Autodesk Inventor part; units mm, degrees
ref_plane "YZ Plane" through (0, 0, 0) normal (1, 0, 0) x (0, 1, 0)
ref_plane "XZ Plane" through (0, 0, 0) normal (0, 1, 0) x (-1, 0, 0)
ref_plane "XY Plane" through (0, 0, 0) normal (0, 0, 1) x (1, 0, 0)
sketch "Sketch1" plane through (0, 0, 0) normal (0, 0, 1) x (1, 0, 0)
  line L0 (6.5024, 2.8448) -> (6.5024, 17.6276)
  line L1 (6.5024, 17.6276) -> (-6.5024, 17.6276)
  line L2 (-6.5024, 2.8448) -> (-6.5024, 17.6276)
  circle A0 centre (0, 0) radius 3.5052 construction
  line L3 (0.1524, -3.5052) -> (-0.1524, -3.5052)
  arc A1 (-6.5024, 2.8448) -> (-0.1524, -3.5052) centre (-0.1524, 2.8448) ccw
  arc A2 (0.1524, -3.5052) -> (6.5024, 2.8448) centre (0.1524, 2.8448) ccw
  circle A3 centre (0, 0) radius 2.1844
  circle A4 centre (0, 0) radius 6.5024 construction
  dimension "d3" = 13.0048
  dimension "d5" = 7.0104
  dimension "d6" = 6.35
  dimension "d7" = 4.3688
  dimension "d10" = 13.0048
  dimension "d11" = 17.6276
extrude "Extrusion1" add sketch "Sketch1" along normal blind 20.32
sketch "Sketch2" plane through (6.5024, 2.8448, 0) normal (1, 0, 0) x (0, 0, -1)
  line L0 (-20.32, 0) -> (-20.32, 14.7828) construction
  line L1 (-20.32, 9.7028) -> (0, 9.7028) construction
  line L2 (0, 14.7828) -> (-20.32, 14.7828) construction
  line L3 (-20.32, 4.9276) -> (0, 4.9276) construction
  line L4 (0, 14.7828) -> (0, 0) construction
  line L5 (0, 0) -> (-20.32, 0) construction
  line L6 (0, -0.6604) -> (-20.32, -0.6604) construction
  line L7 (0, -5.0292) -> (-20.32, -5.0292) construction
  line L8 (0, -0.6604) -> (0, -5.0292) construction
  line L9 (0, -6.35) -> (0, 0) construction
  line L10 (-10.16, 14.7828) -> (-10.16, -6.35) construction
  line L11 (0, -6.35) -> (-20.32, -6.35) construction
  line L12 (-5.9055, 4.9276) -> (-5.9055, -6.35)
  line L13 (-5.9055, -6.35) -> (-10.16, -6.35)
  line L14 (-14.4145, 4.9276) -> (-14.4145, -6.35)
  line L15 (-14.4145, -6.35) -> (-10.16, -6.35)
  line L16 (-10.16, 9.7028) -> (-4.826, 9.7028)
  line L17 (-4.826, 9.7028) -> (-4.826, 4.9276)
  line L18 (-10.16, 9.7028) -> (-15.494, 9.7028)
  line L19 (-15.494, 9.7028) -> (-15.494, 4.9276)
  line L20 (-15.494, 4.9276) -> (-14.4145, 4.9276)
  line L21 (-4.826, 4.9276) -> (-5.9055, 4.9276)
  point P0 (0, -2.8448)
  dimension "d12" = 5.08
  dimension "d14" = 7.7724
  dimension "d15" = 4.2545
  dimension "d16" = 4.2545
extrude "Extrusion2" cut sketch "Sketch2" against normal through all
sketch "Sketch3" plane through (-6.5024, 17.6276, 0) normal (0, 1, 0) x (1, 0, 0)
  line L0 (6.6548, -14.4145) -> (6.6548, -20.32) construction
  line L1 (0, 0) -> (13.0048, 0) construction
  line L2 (6.5024, 0) -> (6.5024, -20.32) construction
  line L3 (13.0048, -20.32) -> (0, -20.32) construction
  line L4 (13.0048, 0) -> (13.0048, -20.32) construction
  line L5 (13.0048, -10.16) -> (0, -10.16) construction
  line L6 (0, 0) -> (0, -20.32) construction
  circle A0 centre (6.5024, -10.16) radius 1.9685 construction
  point P0 (6.5024, 0)
  dimension "d21" = 6.5024
  dimension "d22" = 10.16
  dimension "d23" = 3.937
hole "Hole1" at (0, 17.6276, 10.16) direction (0, -1, 0) diameter 3.937 end through all
sketch "Sketch4" plane through (0, 0, 20.32) normal (0, 0, 1) x (1, 0, 0)
  circle A0 centre (0, 0) radius 3.81
  dimension "d31" = 7.62
extrude "Extrusion3" cut sketch "Sketch4" against normal blind 2.54
sketch "Sketch5" plane through (0, 0, 0) normal (0, 0, -1) x (-1, 0, 0)
  circle A0 centre (0, 0) radius 2.1844 construction
  circle A1 centre (0, 0) radius 4.1275 construction
  line L0 (-4.1275, 0) -> (-2.0638, 3.5745)
  line L1 (-2.0638, 3.5745) -> (2.0637, 3.5745)
  line L2 (2.0637, 3.5745) -> (4.1275, 0)
  line L3 (4.1275, 0) -> (2.0638, -3.5745)
  line L4 (2.0638, -3.5745) -> (-2.0637, -3.5745)
  line L5 (-2.0637, -3.5745) -> (-4.1275, 0)
  dimension "d34" = 8.255
extrude "Extrusion4" cut sketch "Sketch5" against normal blind 2.54
properties part number "omni wheel wheel holder proto"
Here's how the part is built. I have some questions about the finished solid (model axes, mm). A direction names the side the tool comes from. Coordinates: 2 decimals unless noted, no trailing zeros. Order: outer loops, then holes, each group sorted by start corner. A loop starts at its lowest first (then second) coordinate and runs counter-clockwise, first axis right, second up. Notation, with made-up numbers: M 79,41 L 117,41 A8 ccw 117,54 Z; hole C 6.5,79 d2. An arc over 180 degrees is marked long. Answer as a JSON object with one key per item and string values. Group by question number.
(1) Which directions (+Z, -Z, +X, -X, +Y, -Y) give clear straight access to the entire face, cutting with the end or side of a thin tool? Please do faces 1 (the face through (0, 10, 15.494)), 2 (the face through (0.137, 3.808, 19.068)), 3 (the face through (0, 3, 14.414)), 4 (the face through (-3.24, -1.54, 1.25)).
(2) Suppose I cut it at B-B, the plane y = 5. Please give me the cut outline in (x, z), then the cut area to 3 significant figures.
(3) For pin 1 (1.3 mm diameter, centred on x = 0, z = 1.5, fed in from -Y); pin 2 (7 mm diameter, centred on x = 0, y = 0, fed in from -Z); pin 3 (1 mm diameter, centred on x = -5, z = 12, fed in from -Y), each with a flat end and sliding along its axis, tell me the tip position at first contact or that it passes through.
(4) I need wall thicknesses on probe 1 along Z at (x, y) = (-1.75, 11); probe 2 along Z at (x, y) = (-4.75, 7.5); probe 3 along X at (y, z) = (15.45, 10.16). Which ranges of each line are inside material? Lowest first, please.
(5) Suppose I cut it at D-D, the plane y = 1. Please give me the cut outline in (x, z), then the cut area to 3 significant figures.
(6) If we mould it in two halves opening along Z, with no side actions, what happens to faces 5 (the face through (-1.8, -1.5, 2.54)), 6 (the face through (0, 3, 5.906)), 7 (the face through (2, 2, 17.78))? For each: released by +Z, released by -Z, zero draft, split by the parting line, or undercut.
(7) Suppose I cut it at A-A, the plane z = 10.16. Please give me the cut outline in (x, y).
(8) Suppose I cut it at C-C, the plane x = 0.75. Please give me the cut outline in (y, z).
Values found:
{
 "1": {"face 1": "+X, -X", "face 2": "+Z", "face 3": "+X, -X, -Y", "face 4": "-Z"},
 "2": {"outline": "M -6.5,0 L 6.5,0 L 6.5,5.91 L -6.5,5.91 Z; M -6.5,14.41 L 6.5,14.41 L 6.5,20.32 L -6.5,20.32 Z", "area": "154 mm^2"},
 "3": {"pin 1": "stops at y = 3.57", "pin 2": "stops at z = 2.54", "pin 3": "stops at y = 12.55"},
 "4": {"probe 1": "z = 0 to 4.83, 15.49 to 20.32", "probe 2": "z = 0 to 5.91, 14.41 to 20.32", "probe 3": "x = -6.5 to -1.97, 1.97 to 6.5"},
 "5": {"outline": "M -6.23,0 L -3.55,0 L -3.55,2.54 L -1.94,2.54 L -1.94,5.91 L -6.23,5.91 Z; M -6.23,14.41 L -1.94,14.41 L -1.94,17.78 L -3.68,17.78 L -3.68,20.32 L -6.23,20.32 Z; M 1.94,2.54 L 3.55,2.54 L 3.55,0 L 6.23,0 L 6.23,5.91 L 1.94,5.91 Z; M 1.94,14.41 L 6.23,14.41 L 6.23,20.32 L 3.68,20.32 L 3.68,17.78 L 1.94,17.78 Z", "area": "84.3 mm^2"},
 "6": {"face 5": "released by -Z", "face 6": "undercut", "face 7": "released by +Z"},
 "7": {"outline": "M -6.5,12.55 L -1.97,12.55 L -1.97,17.63 L -6.5,17.63 Z; M 1.97,12.55 L 6.5,12.55 L 6.5,17.63 L 1.97,17.63 Z"},
 "8": {"outline": "M -3.48,2.54 L -2.05,2.54 L -2.05,5.91 L -3.48,5.91 Z; M -3.48,14.41 L -2.05,14.41 L -2.05,17.78 L -3.48,17.78 Z; M 2.05,2.54 L 3.57,2.54 L 3.57,0 L 17.63,0 L 17.63,8.34 L 12.55,8.34 L 12.55,4.83 L 7.77,4.83 L 7.77,5.91 L 2.05,5.91 Z; M 2.05,14.41 L 7.77,14.41 L 7.77,15.49 L 12.55,15.49 L 12.55,11.98 L 17.63,11.98 L 17.63,20.32 L 3.74,20.32 L 3.74,17.78 L 2.05,17.78 Z"}
}
